Source: CAD feature listing. Evaluate the final solid. Frame: model axes, mm. A direction names the side the tool comes from. Give positions to 0.01 mm unless a question says otherwise; leave off trailing zeros. Loops run counter-clockwise (first coordinate to the right, second up) from the corner with the lowest first, then second, coordinate; pieces in that order, holes last. Notation, with made-up numbers: (44, 3) -> (49, 3) arc R24 ccw to (49, 21) -> close; hole circle Ø7 at (26, -30.75). An arc over 180 degrees is marked (long way). Return JSON: item names as keys, results as strings. Group by question number.
```python
from build123d import *

# Parameters (mm, degrees)
SKETCH_2_W                   = 8
SKETCH_2_H                   = 24
EXTRUDE_1_DEPTH              = 12
SKETCH_3_W                   = 9.180468112
SKETCH_3_H                   = 14
CUT_EXTRUDE_1_DEPTH          = 40
CHAMFER_1_SIZE               = 1
CHAMFER_1_SIZE2              = 2.747477419
HOLE_WIZARD_M3_1_D           = 3.2
HOLE_WIZARD_M3_1_CBORE_D     = 5.9
HOLE_WIZARD_M3_1_CBORE_DEPTH = 1.6
CUT_EXTRUDE_2_DEPTH          = 1.6
HOLE_WIZARD_1767_D           = 3.2
HOLE_WIZARD_1767_DEPTH       = 24
HOLE_WIZARD_1767_CSINK_D     = 6.6
HOLE_WIZARD_1767_CSINK_ANGLE = 90
HOLE_WIZARD_1767_TIP         = 0.96137699
CHAMFER_2_SIZE               = 1


with BuildPart() as part:
    # 草图2 → 凸台-拉伸1 (new body)
    with BuildSketch(Plane.XY):
        with Locations((97, 93)):
            Rectangle(SKETCH_2_W, SKETCH_2_H)
    extrude(amount=EXTRUDE_1_DEPTH)

    # 草图3 → 切除-拉伸1 (cut)
    with BuildSketch(Plane.ZY.offset(-93)):
        with Locations((8.790234056, 93)):
            Rectangle(SKETCH_3_W, SKETCH_3_H)
    extrude(amount=-CUT_EXTRUDE_1_DEPTH, mode=Mode.SUBTRACT)

    # 倒角1
    chamfer_1_edges = [part.edges().sort_by_distance(p)[0] for p in [
        (97, 86, 4.2),
        (97, 100, 4.2),
    ]]
    chamfer_1_side = [part.faces().sort_by_distance(p)[0] for p in [
        (97, 93, 4.2),
    ]]
    chamfer(chamfer_1_edges, length=CHAMFER_1_SIZE, length2=CHAMFER_1_SIZE2, reference=chamfer_1_side[0])

    # M3 六角头螺栓的柱形沉头孔1 (through all)
    with Locations(Plane(origin=(124.363861944, -131.010130877, 4.2), x_dir=(0, 1, 0), z_dir=(0, 0, 1))):
        with Locations((221.010130877, 27.363861944), (227.010130877, 27.363861944)):
            CounterBoreHole(HOLE_WIZARD_M3_1_D / 2, HOLE_WIZARD_M3_1_CBORE_D / 2, HOLE_WIZARD_M3_1_CBORE_DEPTH)

    # 草图11 → 切除-拉伸2 (cut)
    with BuildSketch(Plane.XY.offset(4.2)):
        with BuildLine():
            Line((94.05, 90), (94.05, 96))
            ThreePointArc((94.05, 96), (97, 98.95), (99.95, 96))
            Line((99.95, 96), (99.95, 90))
            ThreePointArc((99.95, 90), (97, 87.05), (94.05, 90))
        make_face()
    extrude(amount=-CUT_EXTRUDE_2_DEPTH, mode=Mode.SUBTRACT)

    # Hole Wizard 1767
    with Locations(Plane(origin=(124.363861944, 105, -5), x_dir=(-1, 0, 0), z_dir=(0, 1, 0))):
        with Locations((27.363861944, 13.7)):
            CounterSinkHole(HOLE_WIZARD_1767_D / 2, HOLE_WIZARD_1767_CSINK_D / 2, depth=HOLE_WIZARD_1767_DEPTH, counter_sink_angle=HOLE_WIZARD_1767_CSINK_ANGLE)
            with Locations((0, 0, -(HOLE_WIZARD_1767_DEPTH + HOLE_WIZARD_1767_TIP / 2))):  # 118° drill point
                Cone(0, HOLE_WIZARD_1767_D / 2, HOLE_WIZARD_1767_TIP, mode=Mode.SUBTRACT)

    # 倒角2
    chamfer_2_edges = [part.edges().sort_by_distance(p)[0] for p in [
        (93, 102.5, 12),
        (101, 102.5, 12),
        (93, 83.5, 12),
        (101, 83.5, 12),
    ]]
    chamfer(chamfer_2_edges, length=CHAMFER_2_SIZE)


solid = part.part
```
1) Cut plane B-B on y = 83. Return loops of the section in (x, z), then the cut area to 3 significant figures.
2) Cut plane D-D on y = 94.75. Return loops of the section in (x, z), then the cut area to 3 significant figures.
3) Cut plane A-A on z = 3. Return loops of the section in (x, y), then the cut area to 3 significant figures.
4) Reachability of faces 1 (the face through (101, 93, 3)), 2 (the face through (96.944, 99.507, 5.593)), 3 (the face through (94.05, 93, 3)) from +Z, -Z, +X, -X, +Y, -Y: full face, straight path, thin tool, end or side. Return the list, or none.
5) Mould query, pull axis Z, two halves, no side actions, for faces 4 (the face through (95.4, 83.46, 8.77)), 5 (the face through (97, 105, 5)), 6 (the face through (97, 84, 12)). Classes: released by +Z, released by -Z, zero draft, split by the parting line, or undercut.
6) Contact query for flat-ended pins moving along their axis: P1, Ø4, axis at x = 96.5, z = 9.5, coming from the +Y side; P2, Ø3.5, axis at x = 97, y = 96, coming from the +Z side; P3, Ø3, axis at x = 98.5, y = 94.5, coming from the +Z side. Output: stop coordinate, or through.
7) Cut plane C-C on z = 8.7. Return loops of the section in (x, y), then the cut area to 3 significant figures.
8) Material intervals for line 1 (Y direction, x = 97, z = 1.55); line 2 (Y direction, x = 100.75, z = 9.25); line 3 (Z direction, x = 97, y = 101.8), sorted ascending.
Calculated:
{
 "1": {"outline": "(93, 0) -> (101, 0) -> (101, 11) -> (100, 12) -> (94, 12) -> (93, 11) -> close; hole circle Ø3.2 at (97, 8.7)", "area": "87.0 mm2"},
 "2": {"outline": "(93, 0) -> (96, 0) -> (96, 2.6) -> (94.05, 2.6) -> (94.05, 4.2) -> (93, 4.2) -> close; (98, 0) -> (101, 0) -> (101, 4.2) -> (99.95, 4.2) -> (99.95, 2.6) -> (98, 2.6) -> close", "area": "19.0 mm2"},
 "3": {"outline": "(93, 81) -> (101, 81) -> (101, 105) -> (93, 105) -> close; hole (94.05, 90) arc R2.95 ccw to (99.95, 90) -> (99.95, 96) arc R2.95 ccw to (94.05, 96) -> close", "area": "129 mm2"},
 "4": {"face 1": "+Z, -Z, +X, +Y, -Y", "face 2": "+Z, +X, -X", "face 3": "+Z"},
 "5": {"face 4": "undercut", "face 5": "zero draft", "face 6": "released by +Z"},
 "6": {"P1": "y = 104.64", "P2": "z = 2.6", "P3": "z = 4.2"},
 "7": {"outline": "(93, 81) -> (95.4, 81) -> (95.4, 86) -> (93, 86) -> close; (93, 100) -> (95.4, 100) -> (95.4, 103.3) -> (93.7, 105) -> (93, 105) -> close; (98.6, 81) -> (101, 81) -> (101, 86) -> (98.6, 86) -> close; (98.6, 100) -> (101, 100) -> (101, 105) -> (100.3, 105) -> (98.6, 103.3) -> close", "area": "45.1 mm2"},
 "8": {"line 1": "81 to 88.4, 91.6 to 94.4, 97.6 to 105", "line 2": "81 to 86, 100 to 105", "line 3": "0 to 7.1, 10.3 to 12"}
}
